Source: CAD feature listing. Evaluate the final solid. Frame: model axes, mm. A direction names the side the tool comes from. Give positions to 0.01 mm unless a question says otherwise; leave off trailing zeros. Write each loop counter-clockwise with the first axis right and the second up, starting at its lowest first coordinate (ties: lowest second). Pieces come first, ordered by that corner, then holes. Notation, with made-up numbers: (41.5, -10.75) -> (61.5, -10.75) arc R16 cw to (61.5, 3.25) -> close; hole circle Ø5 at (83.5, 50.5). An arc over 180 degrees is marked (long way). Use one line per item in the form item = value. Start each with the question number.
(1) Set-up query: faces 4 (the face through (0.7, -37.15, 76.99)), 5 (the face through (54.9, 11.5, 17.8)). Return all of +Z, -Z, +X, -X, +Y, -Y with unobstructed straight access to the full face (end or side cutting, diameter ignored); none if empty.
(2) First-contact query: P1, Ø2, axis at x = -3.5, y = -23.5, coming from the -Z side; P2, Ø12, axis at y = -3, z = 51.5, coming from the +X side. Flat tips, straight axial feed; report the tip coordinate or a pass-through.
(3) Cut plane B-B, the plane z = 40. Output: boundary loops of the cut face in (x, y).
(4) Cut plane A-A, the plane y = 0. Output: boundary loops of the cut face in (x, z).
(5) Material intervals for line 1 along Z through (x, y) = (54.5, 0); line 2 along X through (y, z) = (-22, 19); line 3 along Z through (x, y) = (54, 8.5), sorted ascending. Write a range as from..to.
(6) Cut plane C-C, the plane x = 53.5. Output: boundary loops of the cut face in (y, z), and give its area (3 significant figures).
(7) Draft query along Y for faces 1 (the face through (55.07, -2.6, 59.83)), 2 (the face through (-1, 40, 35)), 3 (the face through (50, -18, 22)). Return one class per face: pulls with the +Y half, pulls with the -Y half, needs draft (parallel to the pull), parting line crosses it, or undercut.
from build123d import *

# Parameters (mm, degrees)
F0_W     = 100
F0_H     = 80
F1_DEPTH = 80
F2_R     = 10
F3_R     = 25
F4_DEPTH = 10
F5_R     = 20
F6_DEPTH = 10


with BuildPart() as f1:
    # F0 (on Top) → F1 (new body)
    with BuildSketch(Plane.XY):
        Rectangle(F0_W, F0_H)
    extrude(amount=F1_DEPTH)

    # F2
    f2_edges = [f1.edges().sort_by_distance(p)[0] for p in [
        (0, -40, 80),
        (0, 40, 80),
    ]]
    fillet(f2_edges, radius=F2_R)

    # F3 (on face) → F4 (join)
    with BuildSketch(Plane.YZ.offset(50)):
        with Locations((0, 40)):
            Circle(F3_R)
    extrude(amount=F4_DEPTH)

    # F5 (on face) → F6 (cut)
    with BuildSketch(Plane.YZ.offset(60)):
        with Locations((0, 40)):
            Circle(F5_R)
    extrude(amount=-F6_DEPTH, mode=Mode.SUBTRACT)


solid = f1.part
Geometry says:
q1.face_4 = +Z, +X, -X, -Y
q1.face_5 = +X
q2.P1 = 0
q2.P2 = 50
q3.outline = (-50, -40) -> (50, -40) -> (50, -25) -> (60, -25) -> (60, -20) -> (50, -20) -> (50, 20) -> (60, 20) -> (60, 25) -> (50, 25) -> (50, 40) -> (-50, 40) -> close
q4.outline = (-50, 0) -> (50, 0) -> (50, 15) -> (60, 15) -> (60, 20) -> (50, 20) -> (50, 60) -> (60, 60) -> (60, 65) -> (50, 65) -> (50, 80) -> (-50, 80) -> close
q5.line_1 = 15..20, 60..65
q5.line_2 = -50..50
q5.line_3 = 16.49..21.9, 58.1..63.51
q6.outline = circle Ø50 at (0, 40); hole circle Ø40 at (0, 40)
q6.area = 707 mm^2
q7.face_1 = undercut
q7.face_2 = pulls with the +Y half
q7.face_3 = needs draft
